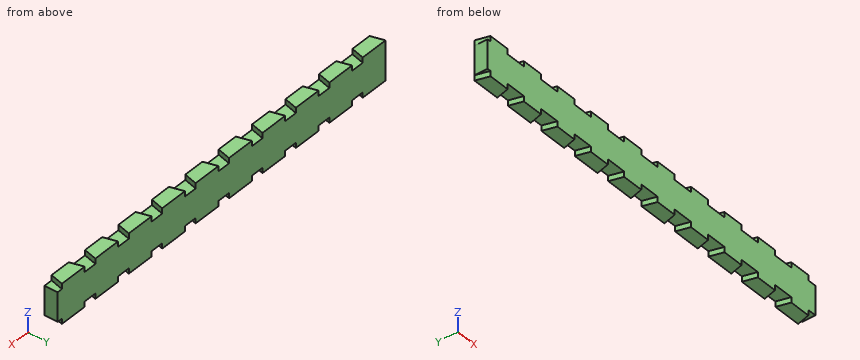
```python
from build123d import *

# Parameters (mm, degrees)
SKETCH2_W            = 1540
SKETCH2_H            = 110
BOSS_EXTRUDE1_DEPTH  = 50
BOSS_EXTRUDE3_DEPTH  = 20
LPATTERN1_COUNT      = 10
LPATTERN1_PITCH      = 157
MIRROR2_COPY_1_DEPTH = 20
MIRROR2_COPY_2_DEPTH = 20
MIRROR2_COPY_3_DEPTH = 20
MIRROR2_COPY_4_DEPTH = 20
MIRROR2_COPY_5_DEPTH = 20
MIRROR2_COPY_6_DEPTH = 20
MIRROR2_COPY_7_DEPTH = 20
MIRROR2_COPY_8_DEPTH = 20
MIRROR2_COPY_9_DEPTH = 20


with BuildPart() as part:
    # Sketch2 → Boss-Extrude1 (new body)
    with BuildSketch(Plane(origin=(0, 0, 0), x_dir=(1, 0, 0), z_dir=(0, 1, 0))):
        Rectangle(SKETCH2_W, SKETCH2_H)
    extrude(amount=BOSS_EXTRUDE1_DEPTH)

    # Sketch4 → Boss-Extrude3 (add)
    with BuildSketch(Plane(origin=(0, 0, -55), x_dir=(-1, 0, 0), z_dir=(0, 0, -1))):
        Polygon((663, 50), (676.397459622, 0), (756.602540378, 0), (770, 50), align=None)
    boss_extrude3 = extrude(amount=BOSS_EXTRUDE3_DEPTH)

    # LPattern1: Boss-Extrude3 ×10
    with Locations(*[(i * LPATTERN1_PITCH, 0, 0) for i in range(1, LPATTERN1_COUNT)]):
        add(boss_extrude3)

    # Mirror2: Boss-Extrude3 across plane
    add(boss_extrude3.mirror(Plane(origin=(0, 0, 0), x_dir=(1, 0, 0), z_dir=(0, 0, -1))))

    # Mirror2 copy 1 sketch → Mirror2 copy 1 (add)
    with BuildSketch(Plane(origin=(157, 0, 55), x_dir=(-1, 0, 0), z_dir=(0, 0, 1))):
        Polygon((663, -50), (676.397459622, 0), (756.602540378, 0), (770, -50), align=None)
    extrude(amount=MIRROR2_COPY_1_DEPTH)

    # Mirror2 copy 2 sketch → Mirror2 copy 2 (add)
    with BuildSketch(Plane(origin=(314, 0, 55), x_dir=(-1, 0, 0), z_dir=(0, 0, 1))):
        Polygon((663, -50), (676.397459622, 0), (756.602540378, 0), (770, -50), align=None)
    extrude(amount=MIRROR2_COPY_2_DEPTH)

    # Mirror2 copy 3 sketch → Mirror2 copy 3 (add)
    with BuildSketch(Plane(origin=(471, 0, 55), x_dir=(-1, 0, 0), z_dir=(0, 0, 1))):
        Polygon((663, -50), (676.397459622, 0), (756.602540378, 0), (770, -50), align=None)
    extrude(amount=MIRROR2_COPY_3_DEPTH)

    # Mirror2 copy 4 sketch → Mirror2 copy 4 (add)
    with BuildSketch(Plane(origin=(628, 0, 55), x_dir=(-1, 0, 0), z_dir=(0, 0, 1))):
        Polygon((663, -50), (676.397459622, 0), (756.602540378, 0), (770, -50), align=None)
    extrude(amount=MIRROR2_COPY_4_DEPTH)

    # Mirror2 copy 5 sketch → Mirror2 copy 5 (add)
    with BuildSketch(Plane(origin=(785, 0, 55), x_dir=(-1, 0, 0), z_dir=(0, 0, 1))):
        Polygon((663, -50), (676.397459622, 0), (756.602540378, 0), (770, -50), align=None)
    extrude(amount=MIRROR2_COPY_5_DEPTH)

    # Mirror2 copy 6 sketch → Mirror2 copy 6 (add)
    with BuildSketch(Plane(origin=(942, 0, 55), x_dir=(-1, 0, 0), z_dir=(0, 0, 1))):
        Polygon((663, -50), (676.397459622, 0), (756.602540378, 0), (770, -50), align=None)
    extrude(amount=MIRROR2_COPY_6_DEPTH)

    # Mirror2 copy 7 sketch → Mirror2 copy 7 (add)
    with BuildSketch(Plane(origin=(1099, 0, 55), x_dir=(-1, 0, 0), z_dir=(0, 0, 1))):
        Polygon((663, -50), (676.397459622, 0), (756.602540378, 0), (770, -50), align=None)
    extrude(amount=MIRROR2_COPY_7_DEPTH)

    # Mirror2 copy 8 sketch → Mirror2 copy 8 (add)
    with BuildSketch(Plane(origin=(1256, 0, 55), x_dir=(-1, 0, 0), z_dir=(0, 0, 1))):
        Polygon((663, -50), (676.397459622, 0), (756.602540378, 0), (770, -50), align=None)
    extrude(amount=MIRROR2_COPY_8_DEPTH)

    # Mirror2 copy 9 sketch → Mirror2 copy 9 (add)
    with BuildSketch(Plane(origin=(1413, 0, 55), x_dir=(-1, 0, 0), z_dir=(0, 0, 1))):
        Polygon((663, -50), (676.397459622, 0), (756.602540378, 0), (770, -50), align=None)
    extrude(amount=MIRROR2_COPY_9_DEPTH)


solid = part.part
```
The model under review builds one solid part; all positions refer to its coordinate system, in mm. Give positions to 0.01 mm unless a question says otherwise; leave off trailing zeros. Write each loop counter-clockwise with the first axis right and the second up, starting at its lowest first coordinate (ties: lowest second). Pieces come first, ordered by that corner, then holes.
(1) For P1, Ø8, axis at x = -342.5, y = 30, coming from the +Z side; P2, Ø16.5, axis at x = 747, y = 20, coming from the -Z side; P3, Ø25, axis at x = -342.5, y = 17, coming from the -Z side, all flat-tipped, find the tip position at first contact; note any pin that passes through.
(2) Consider section A-A, the plane x = -163. Give the boundary of the cut face in (y, z).
(3) To check wall thickness, follow L1, parallel to Z at x = 466, y = 20. State the ranges of the line that lie inside material, in increasing order.
Returned:
1. P1: stops at z = 55
1. P2: stops at z = -75
1. P3: stops at z = -55
2. outline: (0, -55) - (50, -55) - (50, 55) - (0, 55) - close
3. L1: z = -55 to 55
